from build123d import *

# Parameters (mm, degrees)
SKETCH2_R                    = 8
BOSS_EXTRUDE1_DEPTH          = 30
CHAMFER1_SIZE                = 1
CIRPATTERN3_COUNT            = 6
CHAMFER1_OF_CIRPATTERN3_SIZE = 1


with BuildPart() as part:
    # Sketch1 → Revolve1 (revolve)
    with BuildSketch(Plane.XY):
        Polygon((0, 0), (53, 0), (53, 5), (109, 5), (109, 30), (30, 30), (30, 75), (0, 75), align=None)
    revolve(axis=Axis((0, 0, 0), (0, 1, 0)))

    # Sketch2 → Boss-Extrude1 (add)
    with BuildSketch(Plane.XZ.offset(-5)):
        with Locations((0, 81)):
            Circle(SKETCH2_R)
    boss_extrude1 = extrude(amount=BOSS_EXTRUDE1_DEPTH)

    # Chamfer1
    chamfer1_edges = [part.edges().sort_by_distance(p)[0] for p in [
        (-8, -25, 81),
    ]]
    chamfer(chamfer1_edges, length=CHAMFER1_SIZE)

    # CirPattern3: Boss-Extrude1 ×6 about axis
    cirpattern3_axis = Axis((0, 0, 0), (0, 1, 0))
    for i in range(1, CIRPATTERN3_COUNT):
        add(boss_extrude1.rotate(cirpattern3_axis, i * 360 / CIRPATTERN3_COUNT))

    # Chamfer1 of CirPattern3
    chamfer1_of_cirpattern3_edges = [part.edges().sort_by_distance(p)[0] for p in [
        (66.148057707, -25, 47.42820323),
        (74.148057707, -25, -33.57179677),
        (8, -25, -81),
        (-66.148057707, -25, -47.42820323),
        (-74.148057707, -25, 33.57179677),
    ]]
    chamfer(chamfer1_of_cirpattern3_edges, length=CHAMFER1_OF_CIRPATTERN3_SIZE)


solid = part.part
Input: part model. Units: mm. Frame: model coordinates. A direction names the side the tool comes from. Give positions to 0.01 mm unless a question says otherwise; leave off trailing zeros. Order: outer loops, then holes, each group sorted by start corner. A loop starts at its lowest first (then second) coordinate and runs counter-clockwise, first axis right, second up. Notation, with made-up numbers: M 30,13 L 61,13 A10 ccw 61,25 Z; hole C -2,-24 d10. An arc over 180 degrees is marked long. Answer as a JSON object with one key per item and string values.
1. Cut plane A-A, the plane x = 0. Output: boundary loops of the cut face in (y, z).
Result sheet:
{"outline": "M -25,-88 L -24,-89 L 5,-89 L 5,-109 L 30,-109 L 30,-30 L 75,-30 L 75,30 L 30,30 L 30,109 L 5,109 L 5,89 L -24,89 L -25,88 L -25,74 L -24,73 L 5,73 L 5,53 L 0,53 L 0,-53 L 5,-53 L 5,-73 L -24,-73 L -25,-74 Z"}
2. Cut plane B-B, the plane z = 0. Output: boundary loops of the cut face in (x, y), and give its area (3 significant figures).
Result sheet:
{"outline": "M -109,5 L -53,5 L -53,0 L 53,0 L 53,5 L 109,5 L 109,30 L 30,30 L 30,75 L -30,75 L -30,30 L -109,30 Z", "area": "8,680 mm²"}
3. Cut plane C-C, the plane y = 17.5. Output: boundary loops of the cut face in (x, z).
Result sheet:
{"outline": "C 0,0 d218"}
4. Reachability of faces 4 (the cylindrical face through (-1.041, -9.297, 88.932)), 5 (the flat face through (70, -25, -40)), 6 (the flat face through (23, 30, 23)) from +Z, -Z, +X, -X, +Y, -Y: full face, straight path, thin tool, end or side. Return the list, or none.
Result sheet:
{"face 4": "-Y", "face 5": "+Z, -Z, +X, -X, -Y", "face 6": "+Y"}
5. First-contact query: P1, Ø1, axis at x = 76.5, z = 76.5, coming from the -Y side; P2, Ø2, axis at x = -4, y = 1.5, coming from the +Z side; P3, Ø1.5, axis at x = 43, z = -52.5, coming from the +Y side. Flat tips, straight axial feed; report the tip coordinate or a pass-through.
Result sheet:
{"P1": "y = 5", "P2": "z = 88.42", "P3": "y = 30"}
6. Ray query, line 1 (Z direction, x = -2.5, y = -13.5); line 2 (Z direction, x = 1, y = 7); line 3 (Y direction, x = 91.5, z = 56.5). Return the intervals inside material, ascending. Write a range as [from, to].
Result sheet:
{"line 1": "[-88.6, -73.4], [73.4, 88.6]", "line 2": "[-109, 109]", "line 3": "[5, 30]"}
7. Cut plane D-D, the plane z = 40.5. Output: boundary loops of the cut face in (x, y).
Result sheet:
{"outline": "M -101.2,5 L -78.15,5 L -78.15,-24 L -77.15,-25 L -63.15,-25 L -62.15,-24 L -62.15,5 L -34.19,5 L -34.19,0 L 34.19,0 L 34.19,5 L 62.15,5 L 62.15,-24 L 63.15,-25 L 77.15,-25 L 78.15,-24 L 78.15,5 L 101.2,5 L 101.2,30 L -101.2,30 Z"}
8. Pull-direction query (Z, two-part tool) for faces 1 (the flat face through (-70, -25, -41)), 2 (the cylindrical face through (62.156, -9.297, -40.148)), 3 (the cylindrical face through (-86.5, 17.68, 66.32)); classes: +Z half, -Z half, draft (parallel to the pull), parting line (faces both ways), or undercut.
Result sheet:
{"face 1": "draft", "face 2": "undercut", "face 3": "parting line"}
